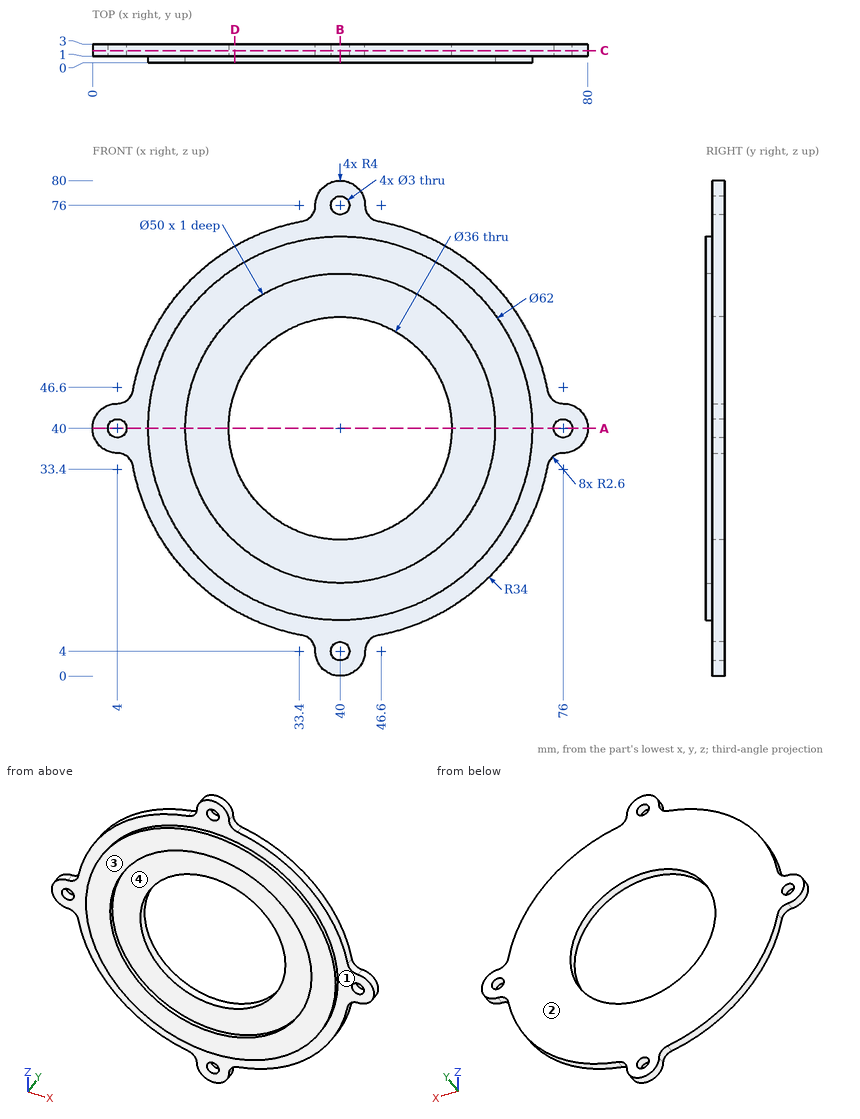
The drawing under review shows one solid part. Ordinate dimensions are in mm from its lowest x, y, z. A direction names the side the tool comes from. Round coordinates to 2 decimals unless told otherwise and drop trailing zeros. Write each loop counter-clockwise with the first axis right and the second up, starting at its lowest first coordinate (ties: lowest second). Pieces come first, ordered by that corner, then holes. Notation, with made-up numbers: (-37.75, 72) - (0.25, 72) arc R9 cw to (0.25, 78) - close; hole circle Ø10 at (87.25, 3). An arc over 180 degrees is marked (long way). Use one line per item in the form item = value.
Q1. Draft analysis for pull direction Z (two halves, no side actions). For the marked faces 3 and 4, state which applies: +Z half, -Z half, draft (parallel to the pull), parting line (faces both ways), or undercut.
Answer key:
face_3 = draft
face_4 = undercut
Q2. Insertion check: pin 1 Ø1 at (x, z) = (22.5, 13.5) entering from -Y; pin 2 Ø1.5 at (x, y) = (20.5, 1.5) entering from -Z. Each pin has a flat end and moves straight along its axis. Give the tip position at first contact, or say it passes through.
Answer key:
pin_1 = 1
pin_2 = 11.64
Q3. For line 1 (X direction, y = 1.45, z = 40); line 2 (Z direction, x = 4, y = 2.5), list the stretches that pass through material, from the lowest coordinate up. Write a range as [from, to].
Answer key:
line_1 = [0, 2.5], [5.5, 22], [58, 74.5], [77.5, 80]
line_2 = [36, 38.5], [41.5, 44]
Q4. Consider section B-B (x = 40). State the section outline as (y, z) points.
Answer key:
outline = (0, 9) - (1, 9) - (1, 5.5) - (3, 5.5) - (3, 22) - (1, 22) - (1, 15) - (0, 15) - close; (0, 65) - (1, 65) - (1, 58) - (3, 58) - (3, 74.5) - (1, 74.5) - (1, 71) - (0, 71) - close; (1, 0) - (3, 0) - (3, 2.5) - (1, 2.5) - close; (1, 77.5) - (3, 77.5) - (3, 80) - (1, 80) - close
Q5. Consider section D-D (x = 23). State the section outline as (y, z) points.
Answer key:
outline = (0, 14.08) - (1, 14.08) - (1, 10.56) - (3, 10.56) - (3, 34.08) - (1, 34.08) - (1, 21.67) - (0, 21.67) - close; (0, 58.33) - (1, 58.33) - (1, 45.92) - (3, 45.92) - (3, 69.44) - (1, 69.44) - (1, 65.92) - (0, 65.92) - close
Q6. Tool access review of the marked faces 1 and 2: name each direction out of +Z, -Z, +X, -X, +Y, -Y from which nothing blocks a thin tool from reaching the whole face with its end or side.
Answer key:
face_1 = -Y
face_2 = +Z, -Z, +X, -X, +Y
Q7. Consider section A-A (z = 40). State the section outline as (x, y) points, and give its area (3 significant figures).
Answer key:
outline = (0, 1) - (2.5, 1) - (2.5, 3) - (0, 3) - close; (5.5, 1) - (9, 1) - (9, 0) - (15, 0) - (15, 1) - (22, 1) - (22, 3) - (5.5, 3) - close; (58, 1) - (65, 1) - (65, 0) - (71, 0) - (71, 1) - (74.5, 1) - (74.5, 3) - (58, 3) - close; (77.5, 1) - (80, 1) - (80, 3) - (77.5, 3) - close
area = 88.0 mm2
Q8. Consider section C-C (y = 1.95). State the section outline as (x, z) points, and give its area (3 significant figures).
Answer key:
outline = (4, 36) arc R2.6 cw to (6.56, 33.87) arc R34 ccw to (33.87, 6.56) arc R2.6 cw to (36, 4) arc R4 ccw to (44, 4) arc R2.6 cw to (46.13, 6.56) arc R34 ccw to (73.44, 33.87) arc R2.6 cw to (76, 36) arc R4 ccw to (76, 44) arc R2.6 cw to (73.44, 46.13) arc R34 ccw to (46.13, 73.44) arc R2.6 cw to (44, 76) arc R4 ccw to (36, 76) arc R2.6 cw to (33.87, 73.44) arc R34 ccw to (6.56, 46.13) arc R2.6 cw to (4, 44) arc R4 ccw to start; hole circle Ø3 at (4, 40); hole circle Ø36 at (40, 40); hole circle Ø3 at (40, 4); hole circle Ø3 at (40, 76); hole circle Ø3 at (76, 40)
area = 2,760 mm2
